Source: three-view drawing plus pictorial views. Frame: mm from the lowest corner of the part. A direction names the side the tool comes from. Round coordinates to 2 decimals unless told otherwise and drop trailing zeros. Write each loop counter-clockwise with the first axis right and the second up, starting at its lowest first coordinate (ties: lowest second). Pieces come first, ordered by that corner, then holes. Notation, with made-up numbers: M 56.5,-1 L 111.5,-1 A18 cw 111.5,29 Z; hole C -33,71 d7. An arc over 180 degrees is marked long. Answer as CSV lines item,"result". Start each with the question number.
Q1. Section query D-D on z = 55. Output: boundary loops of the cut face in (x, y), and give its area (3 significant figures).
Q2. First-contact query: pin 1 (1.5 mm diameter, centred on x = 29.5, z = 41, fed in from +Y); pin 2 (5 mm diameter, centred on y = 4, z = 51.5, fed in from -X); pin 3 (5 mm diameter, centred on y = 17, z = 48, fed in from -X). Flat tips, straight axial feed; report the tip coordinate or a pass-through.
Q3. Reachability of the marked faces 1, 2 and 3 from +Z, -Z, +X, -X, +Y, -Y: full face, straight path, thin tool, end or side. Return the list, or none.
Q4. Section query B-B on y = 52. Output: boundary loops of the cut face in (x, z), and give its area (3 significant figures).
Q5. Section query A-A on z = 44. Output: boundary loops of the cut face in (x, y).
Q6. Section query C-C on x = 36. Output: boundary loops of the cut face in (y, z), and give its area (3 significant figures).
Q7. Ray query, probe 1 along X at (y, z) = (42, 36); probe 2 along X at (y, z) = (15, 34); probe 3 along Z at (x, y) = (57.5, 41). Return the intervals inside material, ascending.
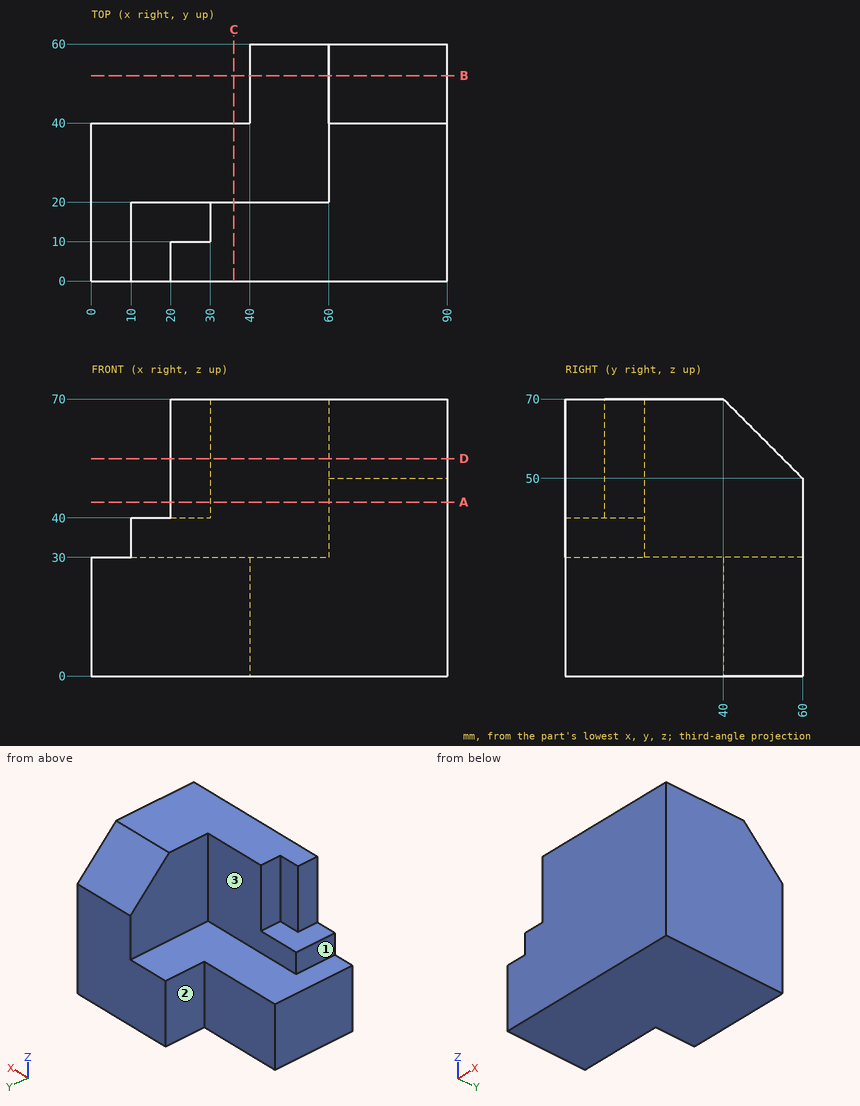
Entries:
1,outline,"M 20,0 L 90,0 L 90,55 L 60,55 L 60,20 L 30,20 L 30,10 L 20,10 Z"
1,area,"2,350 mm^2"
2,pin 1,"stops at y = 20"
2,pin 2,"stops at x = 20"
2,pin 3,"stops at x = 30"
3,face 1,"+Z, -X, +Y, -Y"
3,face 2,"+Z, -Z, -X, +Y"
3,face 3,"+Z, -X, +Y"
4,outline,"M 40,0 L 90,0 L 90,58 L 60,58 L 60,30 L 40,30 Z"
4,area,"2,340 mm^2"
5,outline,"M 20,0 L 90,0 L 90,60 L 60,60 L 60,20 L 30,20 L 30,10 L 20,10 Z"
6,outline,"M 0,0 L 40,0 L 40,30 L 20,30 L 20,70 L 0,70 Z"
6,area,"2,000 mm^2"
7,probe 1,"x = 60 to 90"
7,probe 2,"x = 10 to 90"
7,probe 3,"z = 0 to 30"
